Here's the drawing with two shaded views (mm, measured from the low corner). I have some questions. A direction names the side the tool comes from. Give positions to 0.01 mm unless a question says otherwise; leave off trailing zeros. Loops run counter-clockwise (first coordinate to the right, second up) from the corner with the lowest first, then second, coordinate; pieces in that order, holes last.
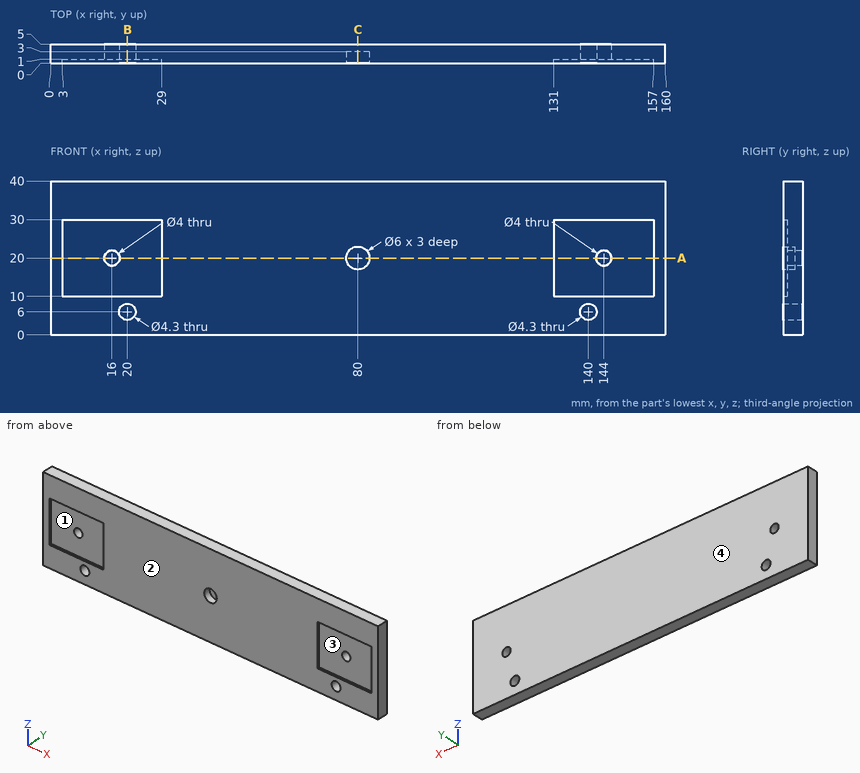
(1) Please list where these lines run through material, in increasing order: probe 1 along X at (y, z) = (3.5, 20); probe 2 along X at (y, z) = (3.8, 6); probe 3 along X at (y, z) = (1.4, 20).
Returned:
probe 1: x = 0 to 14, 18 to 142, 146 to 160
probe 2: x = 0 to 17.85, 22.15 to 137.85, 142.15 to 160
probe 3: x = 0 to 14, 18 to 77, 83 to 142, 146 to 160
(2) Will this pin go through, and if not, where does the flat tip stop? P1, Ø6.5, axis at x = 16, z = 20, coming from the -Y side.
Returned:
P1: stops at y = 1
(3) Thinking about a two-plate mould opening in Z: for the marked faces 1 and 2, which applies, pulls with the +Z half, pulls with the -Z half, needs draft (parallel to the pull), parting line crosses it, or undercut?
Returned:
face 1: undercut
face 2: needs draft
(4) Which directions (+Z, -Z, +X, -X, +Y, -Y) give clear straight access to the entire face, cutting with the end or side of a thin tool? Please do the marked faces 3 and 4.
Returned:
face 3: -Y
face 4: +Z, -Z, +X, -X, +Y
(5) Suppose I cut it at A-A on z = 20. List the corners of the cut face in (x, y) for me.
Returned:
outline: (0, 0) - (3, 0) - (3, 1) - (14, 1) - (14, 5) - (0, 5) - close; (18, 1) - (29, 1) - (29, 0) - (77, 0) - (77, 3) - (83, 3) - (83, 0) - (131, 0) - (131, 1) - (142, 1) - (142, 5) - (18, 5) - close; (146, 1) - (157, 1) - (157, 0) - (160, 0) - (160, 5) - (146, 5) - close
(6) Suppose I cut it at B-B on x = 20. List the corners of the cut face in (y, z) for me.
Returned:
outline: (0, 0) - (5, 0) - (5, 3.85) - (0, 3.85) - close; (0, 8.15) - (5, 8.15) - (5, 40) - (0, 40) - (0, 30) - (1, 30) - (1, 10) - (0, 10) - close
(7) Suppose I cut it at C-C on x = 80. List the corners of the cut face in (y, z) for me.
Returned:
outline: (0, 0) - (5, 0) - (5, 40) - (0, 40) - (0, 23) - (3, 23) - (3, 17) - (0, 17) - close
